Build history of the part. All positions in model axes, mm. A direction names the side the tool comes from. Coordinates: 2 decimals unless noted, no trailing zeros. Write each loop counter-clockwise with the first axis right and the second up, starting at its lowest first coordinate (ties: lowest second). Pieces come first, ordered by that corner, then holes.
```python
from build123d import *

# Parameters (mm, degrees)
F2_SIZE  = 3
F3_R     = 3
F4_DEPTH = 50
F5_R     = 3
F6_DEPTH = 50
F7_R     = 5
F8_DEPTH = 10


with BuildPart() as f1:
    # F0 (on Right) → F1 (revolve)
    with BuildSketch(Plane.YZ):
        Polygon((-50, 0), (-16, 0), (-16, 15), (-20, 15), (-20, 20), (-16, 20), (-16, 40), (-20, 50), (-20, 90), (-25, 90), (-25, 75), (-30, 75), (-30, 65), (-27, 65), (-27, 60), (-30, 60), (-30, 10), (-50, 10), align=None)
    revolve(axis=Axis((0, 0, 45), (0, 0, 1)))

    # F2
    f2_edges = [f1.edges().sort_by_distance(p)[0] for p in [
        (0, 16, 0),
    ]]
    chamfer(f2_edges, length=F2_SIZE)

    # F3 (on Front) → F4 (cut, symmetric)
    with BuildSketch(Plane.XZ):
        with Locations((0, 30)):
            Circle(F3_R)
    extrude(amount=F4_DEPTH, both=True, mode=Mode.SUBTRACT)

    # F5 (on Right) → F6 (cut, symmetric)
    with BuildSketch(Plane.YZ):
        with Locations((0, 30)):
            Circle(F5_R)
    extrude(amount=F6_DEPTH, both=True, mode=Mode.SUBTRACT)

    # F7 (on face) → F8 (cut, through all)
    with BuildSketch(Plane.XY.offset(10)):
        with Locations((0, -40)):
            Circle(F7_R)
        with Locations((40, 0)):
            Circle(F7_R)
        with Locations((0, 40)):
            Circle(F7_R)
        with Locations((-40, 0)):
            Circle(F7_R)
    extrude(amount=-F8_DEPTH, mode=Mode.SUBTRACT)


solid = f1.part
```
1. Saw through at D-D on y = 0. State how many separate pieces and enclosed holes the cut face has, plus the area to 3 significant figures.
Computed values:
separate pieces: 6
enclosed holes: 0
area: 1,960 mm2
2. Saw through at C-C on x = 22. List the corners of the cut face in (y, z).
Computed values:
outline: (-44.9, 0) - (44.9, 0) - (44.9, 10) - (20.4, 10) - (20.4, 60) - (15.65, 60) - (15.65, 65) - (20.4, 65) - (20.4, 75) - (11.87, 75) - (11.87, 90) - (-11.87, 90) - (-11.87, 75) - (-20.4, 75) - (-20.4, 65) - (-15.65, 65) - (-15.65, 60) - (-20.4, 60) - (-20.4, 10) - (-44.9, 10) - close; hole circle Ø6 at (0, 30)
3. 3-axis set-ups, long thin cutter, end or side, ignore diameter. For faces 1 (the face through (-19.524, 4.336, 17.535)), 2 (the face through (1.32, 29.97, 69.93)), 3 (the face through (-22, 1, 0)): which of +Z, -Z, +X, -X, +Y, -Y reach the whole face in a straight line?
Computed values:
face 1: none
face 2: +Z
face 3: -Z, +X, -X, +Y, -Y
4. Flat gauge pins, fed straight in: pin 1 (2 mm diameter, centred on x = 13, y = 23.5, fed in from +Z); pin 2 (18 mm diameter, centred on x = -3.5, y = 10, fed in from +Z); pin 3 (11.5 mm diameter, centred on x = 0, y = -40, fed in from +Z). Where does each tip first touch, or does it go through?
Computed values:
pin 1: stops at z = 75
pin 2: stops at z = 48.99
pin 3: stops at z = 10
5. Mould opens along Z. For faces 4 (the face through (13.43, -8.98, 15)), 5 (the face through (25, -7, 75)), 6 (the face through (-2.21, 22.76, 32.03)), 7 (the face through (15.02, -47.69, 4.93)) say: +Z half, -Z half, draft (parallel to the pull), parting line (faces both ways), or undercut.
Computed values:
face 4: undercut
face 5: +Z half
face 6: undercut
face 7: draft
6. Probe line 1 along Y through (x, z) = (-0.5, 69); line 2 along Y through (x, z) = (1, 77); line 3 along Z through (x, y) = (-21.5, 43). List the from-to ranges inside material, lowest first.
Computed values:
line 1: y = -30 to -19.99, 19.99 to 30
line 2: y = -24.98 to -19.97, 19.97 to 24.98
line 3: z = 0 to 10
7. Saw through at A-A on x = 40. List the corners of the cut face in (y, z), plus the area to 3 significant figures.
Computed values:
outline: (-30, 0) - (-5, 0) - (-5, 10) - (-30, 10) - close; (5, 0) - (30, 0) - (30, 10) - (5, 10) - close
area: 500 mm2
